Check sheet for the modelled part. Datum: model origin and axes. Units: mm. Face numbers are marked on the shaded views. A direction names the side the tool comes from. Give positions to 0.01 mm unless a question says otherwise; leave off trailing zeros. Loops run counter-clockwise (first coordinate to the right, second up) from the corner with the lowest first, then second, coordinate; pieces in that order, holes last. Notation, with made-up numbers: (-30, 38) - (-4, 38) arc R13 cw to (-4, 62) - close; hole circle Ø6 at (73.25, 4). An arc over 180 degrees is marked (long way). Use CSV: the item, a comma, the result in double quotes.
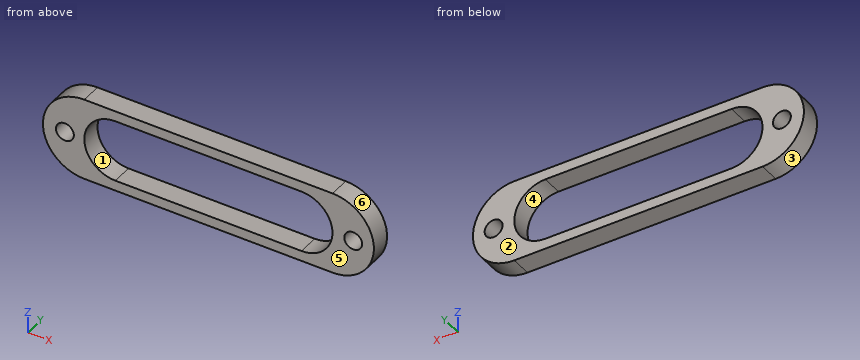
from build123d import *

# Parameters (mm, degrees)
BOSS_EXTRUDE1_DEPTH  = 6.35
M5_CLEARANCE_HOLE1_D = 5.5


with BuildPart() as part:
    # Sketch2 → Boss-Extrude1 (new body)
    with BuildSketch(Plane(origin=(0, 0, 0), x_dir=(1, 0, 0), z_dir=(0, 1, 0))):
        with BuildLine():
            Line((0, 12.7), (76.2, 12.7))
            ThreePointArc((76.2, 12.7), (88.9, 0), (76.2, -12.7))
            Line((76.2, -12.7), (0, -12.7))
            ThreePointArc((0, -12.7), (-12.7, 0), (0, 12.7))
        make_face()
        with BuildLine():
            Line((9.525, 9.525), (66.675, 9.525))
            ThreePointArc((66.675, 9.525), (76.2, 0), (66.675, -9.525))
            Line((66.675, -9.525), (9.525, -9.525))
            ThreePointArc((9.525, -9.525), (0, 0), (9.525, 9.525))
        make_face(mode=Mode.SUBTRACT)
    extrude(amount=BOSS_EXTRUDE1_DEPTH)

    # M5 Clearance Hole1 (through all)
    with Locations(Plane(origin=(0, 6.35, 0), x_dir=(1, 0, 0), z_dir=(0, 1, 0))):
        with Locations((-5.950002807, 0), (82.55, 0)):
            Hole(M5_CLEARANCE_HOLE1_D / 2)


solid = part.part
1. Sectioned sample at A-A, the plane x = 17.5. Record the boundary of the cut face in (y, z) (3 decimals), and give its area (3 significant figures).
Completed:
outline,"(0, -12.7) - (6.35, -12.7) - (6.35, -9.525) - (0, -9.525) - close; (0, 9.525) - (6.35, 9.525) - (6.35, 12.7) - (0, 12.7) - close"
area,"40.3 mm²"
2. Sectioned sample at B-B, the plane z = 0. Record the boundary of the cut face in (x, y), and give its area (3 significant figures).
Completed:
outline,"(-12.7, 0) - (-8.7, 0) - (-8.7, 6.35) - (-12.7, 6.35) - close; (-3.2, 0) - (0, 0) - (0, 6.35) - (-3.2, 6.35) - close; (76.2, 0) - (79.8, 0) - (79.8, 6.35) - (76.2, 6.35) - close; (85.3, 0) - (88.9, 0) - (88.9, 6.35) - (85.3, 6.35) - close"
area,"91.4 mm²"
3. Sectioned sample at C-C, the plane y = 2. Record the boundary of the cut face in (x, z) (3 decimals), and give its area (3 significant figures).
Completed:
outline,"(0, -12.7) - (76.2, -12.7) arc R12.7 ccw to (76.2, 12.7) - (0, 12.7) arc R12.7 ccw to start; hole circle Ø5.5 at (-5.95, 0); hole (9.525, -9.525) - (66.675, -9.525) arc R9.525 ccw to (66.675, 9.525) - (9.525, 9.525) arc R9.525 ccw to start; hole circle Ø5.5 at (82.55, 0)"
area,"1,020 mm²"
4. Scan lines: line 1 along X through (y, z) = (3.25, 0.25); line 2 along Z through (x, y) = (48.5, 3.25) (3 decimals); line 3 along Z through (x, y) = (82.55, 4). Record each from-to range of solid material in increasing order.
Completed:
line 1,"x = -12.7 to -8.69, -3.21 to 0, 76.2 to 79.81, 85.29 to 88.9"
line 2,"z = -12.7 to -9.525, 9.525 to 12.7"
line 3,"z = -11 to -2.75, 2.75 to 11"
5. Go/stop test with flat-tipped pins: pin 1 Ø2 at (y, z) = (3, -4) entering from -X; pin 2 Ø4.5 at (x, z) = (-5.95, 0) entering from +Y; pin 3 Ø1 at (y, z) = (1, 3) entering from -X. Record where each tip stops, or that it passes through.
Completed:
pin 1,"stops at x = -12.34"
pin 2,"passes through"
pin 3,"stops at x = -12.45"
6. Sectioned sample at D-D, the plane z = 8.25. Record the boundary of the cut face in (x, y).
Completed:
outline,"(-9.66, 0) - (4.76, 0) - (4.76, 6.35) - (-9.66, 6.35) - close; (71.44, 0) - (85.86, 0) - (85.86, 6.35) - (71.44, 6.35) - close"
7. Set-up check for the marked faces 1 and 2: record each of +Z, -Z, +X, -X, +Y, -Y from which the full face is reachable in a straight line by a thin tool's end or side.
Completed:
face 1,"+Y, -Y"
face 2,"+Z, -Z, +X, -X, +Y"
8. Release check for a two-part mould opening along X. For the marked faces 3, 4, 5 and 6 record: released by +X, released by -X, zero draft, split by the parting line, or undercut.
Completed:
face 3,"released by -X"
face 4,"undercut"
face 5,"zero draft"
face 6,"released by +X"
